Could you check a few things on this model? Use its own coordinates, in mm. Face numbers are marked on the shaded views. A direction names the side the tool comes from. Round coordinates to 2 decimals unless told otherwise and drop trailing zeros. Order: outer loops, then holes, each group sorted by start corner. A loop starts at its lowest first (then second) coordinate and runs counter-clockwise, first axis right, second up. Notation, with made-up numbers: (-11, 15) -> (19, 15) arc R16 ccw to (19, 43) -> close; hole circle Ø4 at (-0.5, 69.5). An arc over 180 degrees is marked (long way). Put each result on its own line as item: value. Start each with the question number.
Autodesk Inventor part; units mm, degrees
ref_plane "Work Plane1" through (29, 0, 0) normal (0, -1, 0) x (1, 0, 0)
ref_plane "YZ Plane" through (0, 0, 0) normal (1, 0, 0) x (0, 1, 0)
ref_plane "XZ Plane" through (0, 0, 0) normal (0, 1, 0) x (-1, 0, 0)
sketch "Sketch1" plane through (0, 0, 0) normal (0, 0, 1) x (1, 0, 0)
  line L0 (0.0567, 0) -> (6, 0)
  line L1 (6, 0) -> (6, 1.5)
  line L2 (6, 1.5) -> (1, 1.5)
  line L3 (1, 1.5) -> (0.6932, 1.5)
  line L4 (0.6932, 1.5) -> (0, 1.5)
  line L5 (0, 1.5) -> (0, 2.85)
  line L6 (0, 2.85) -> (-1.65, 2.85)
  line L7 (-1.65, 2.85) -> (-1.65, 1.1547)
  line L8 (-1.65, 1.1547) -> (-0.61, 1.1547)
  line L9 (-0.61, 1.1547) -> (0.0567, 0)
  line L10 (-3.18, 0) -> (7.53, 0)
  line L11 (0, -0.57) -> (0, 3.42)
  line L12 (1, 1.5) -> (0, 1.5) construction
  dimension "d1" = 5
  dimension "d2" = 0.3068
  dimension "d3" = 1.65
  dimension "d4" = 1.04
  dimension "d5" = 60
  dimension "d6" = 3
  dimension "d7" = 3
  dimension "d8" = 2.3094
  dimension "d9" = 5.7
  dimension "d26" = 6
revolve "Body" add sketch "Sketch1" angle 360 about axis through (0.0567, 0, 0) along (1, 0, 0) contours L9 L11 L4 L3 L2 L1 L0 | L9 L8 L7 L6 L5 L11
sketch "Sketch2" plane through (-1.65, 0, 0) normal (-1, 0, 0) x (0, 0, 1)
  circle A0 centre (0, 0) radius 1.1547
  line L0 (0, -3.99) -> (0, 3.99)
  line L1 (-3.99, 0) -> (3.99, 0)
  line L2 (1.1547, 0) -> (0.5774, -1)
  line L3 (0.5774, -1) -> (-0.5774, -1)
  line L4 (-0.5774, -1) -> (-1.1547, 0)
  line L5 (-1.1547, 0) -> (-0.5774, 1)
  line L6 (-0.5774, 1) -> (0.5774, 1)
  line L7 (0.5774, 1) -> (1.1547, 0)
extrude "Slot" add sketch "Sketch2" against normal up to next contours L7 A0 | A0 L2 | L6 L0 A0 | A0 L0 L3 | L0 L6 A0 | A0 L3 L0 | L4 A0 | A0 L5
fillet "Fillet1" radius 1.45 1 edges at (-1.65, -2.85, 0)
thread "Thread"
chamfer "Chamfer1" distance 0.3067 distance2 0.3067 1 edges at (6, -1.5, 0) measured on face at (6, 0.3952, 0.0397)
ref_plane "Work Plane1" through (29, 0, 0) normal (0, -1, 0) x (1, 0, 0)
fillet "Fillet2" radius 0.1 1 edges at (0, -1.5, 0)
equation "\"d1\" = GEL"
equation "\"d3\" = KOH"
equation "\"d4\" = INTI"
equation "\"d6\" = GD"
equation "\"d7\" = BDM"
equation "\"d8\" = 1.1547 * SW"
equation "\"d9\" = KOD"
equation "\"d26\" = NLG"
equation "\"d30\" = R"
equation "\"d17\" = RR"
equation "\"d13\" = GEL"
equation "\"d15\" = -0.5 * SPD + 0.5 * GD"
equation "\"d16\" = GUL"
equation "\"GD\" = 3"
equation "\"NLG\" = 6"
equation "\"GEL\" = 5"
equation "\"KOD\" = 5.7"
equation "\"KOH\" = 1.65"
equation "\"INTI\" = 1.04"
equation "\"GAL\" = 0.61345 * PTC"
equation "\"GUL\" = 0.61345 * PTC"
equation "\"BDM\" = 3"
equation "\"SW\" = 2"
equation "\"RR\" = 1.45"
equation "\"SPD\" = NND - 1.2269 * PTC"
equation "\"R\" = 0.1"
equation "\"TOA\" = 30deg"
equation "\"GD1\" = THREADDIA - 1.2269 * PTC"
equation "\"THREADDIA\" = 3"
equation "\"PTC\" = 0.5"
equation "\"NND\" = 3"
equation "\"KOH1\" = 0.2"
equation "\"E0\" = 2.31"
properties part number "Screw GB/T 70.2 M3 X 6" material "Steel, Mild"
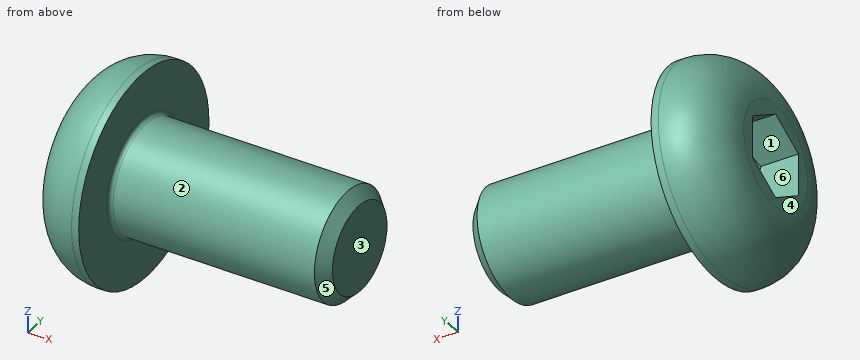
1. Thinking about a two-plate mould opening in Z: for the marked faces 4, 5 and 6, which applies, +Z half, -Z half, draft (parallel to the pull), parting line (faces both ways), or undercut?
2. Which directions (+Z, -Z, +X, -X, +Y, -Y) give clear straight access to the entire face, cutting with the end or side of a thin tool? Please do the marked faces 1, 2 and 3.
3. If we section it at A-A, the plane x = 4: Please give me the cut outline in (y, z), then the cut area to 3 significant figures.
4. I need wall thicknesses on L1, parallel to X at y = 1.75, z = 0.35; L2, parallel to X at y = 0.95, z = -1.8; L3, parallel to Z at x = 1.25, y = 1.1. Which ranges of each line are inside material? Lowest first, please.
5. For pin 1 Ø1 at (x, y) = (1.5, -1) entering from +Z; pin 2 Ø1.2 at (x, z) = (-1, 0) entering from +Y; pin 3 Ø2 at (x, z) = (5, -1.5) entering from -Y, each with a flat end and sliding along its axis, tell me the tip position at first contact or that it passes through.
Results below:
1. face 4: draft
1. face 5: parting line
1. face 6: undercut
2. face 1: -X
2. face 2: +X
2. face 3: +Z, -Z, +X, +Y, -Y
3. outline: circle Ø3 at (0, 0)
3. area: 7.07 mm2
4. L1: -1.6 to 0
4. L2: -1.5 to 0
4. L3: -1.02 to 1.02
5. pin 1: z = 1.41
5. pin 2: y = 2.84
5. pin 3: y = -1.41
